Read the model definition and answer for the solid it produces. Units are mm, in the model's axes. A direction names the side the tool comes from. Coordinates: 2 decimals unless noted, no trailing zeros. Write each loop counter-clockwise with the first axis right and the second up, starting at its lowest first coordinate (ties: lowest second). Pieces come first, ordered by that corner, then holes. Notation, with made-up numbers: (11.25, 19) -> (31.25, 19) arc R24 ccw to (31.25, 55) -> close; hole circle Ø4 at (6, 33.5). An arc over 180 degrees is marked (long way). One line per item, written item: value. Start each with the question number.
1. For a pull along Y with two mould halves and no side action, classify faces 6 (the cylindrical face through (0, -15, 0)), 7 (the flat face through (0, -16.75, 0)), 8 (the flat face through (2, -7, -1.5)) as pulls with the +Y half, pulls with the -Y half, needs draft (parallel to the pull), parting line crosses it, or undercut.
2. For faces 1 (the flat face through (-5, 1.2, 1.14)), 2 (the cylindrical face through (0, -1.5, 0)), 3 (the cylindrical face through (7.03, 0.07, 1.5)), 4 (the flat face through (5, -1.2, -1.14)), 5 (the flat face through (-4, -9, 0)), determine the directions among +Z, -Z, +X, -X, +Y, -Y from which every point of the face is accessible in a straight line to the end or side of a thin tool.
3. Given P1, Ø3, axis at x = 7.5, y = -2, coming from the +Z side; P2, Ø2, axis at x = 0, y = -9.5, coming from the +Z side; P3, Ø1.5, axis at y = -12, z = -1, coming from the -X side, each flat-ended and moving along its own axis, determine where each tip first touches the part or whether it passes through.
4. Find section A-A, the plane x = 0. Write down the section's boundary in (y, z), and give its area (4 significant figures).
5. Consider line 1 along X through (y, z) = (-10.25, -0.2); line 2 along X through (y, z) = (-14, 1.05); line 3 along Y through (x, z) = (0.5, -0.3). Determine where each line is inside the solid, lowest interval first.
6. Find section B-B, the plane y = -12.25. Write down the section's boundary in (x, z), and give its area (3 significant figures).
```python
from build123d import *

# Parameters (mm, degrees)
BOSS_EXTRU_1_DEPTH = 1.5
ESQUISSE3_R        = 1.5
BOSS_EXTRU_2_DEPTH = 10


with BuildPart() as part:
    # Esquisse1 → Boss.-Extru.1 (new, symmetric)
    with BuildSketch(Plane.XY):
        with BuildLine():
            Line((-5, -1.5), (-4.585786438, -1.914213562))
            ThreePointArc((-4.585786438, -1.914213562), (-4.152240935, -2.56306026), (-4, -3.328427125))
            Line((-4, -3.328427125), (-4, -14.75))
            ThreePointArc((-4, -14.75), (-3.414213562, -16.164213562), (-2, -16.75))
            Line((-2, -16.75), (2, -16.75))
            ThreePointArc((2, -16.75), (3.414213562, -16.164213562), (4, -14.75))
            Line((4, -14.75), (4, -3.328427125))
            ThreePointArc((4, -3.328427125), (4.152240935, -2.56306026), (4.585786438, -1.914213562))
            Line((4.585786438, -1.914213562), (5, -1.5))
            Line((5, -1.5), (5, 1.5))
            Line((5, 1.5), (-5, 1.5))
            Line((-5, 1.5), (-5, -1.5))
        make_face()
        with BuildLine():
            Line((1.75, -3.25), (1.75, -13.25))
            ThreePointArc((1.75, -13.25), (0, -15), (-1.75, -13.25))
            Line((-1.75, -13.25), (-1.75, -3.25))
            ThreePointArc((-1.75, -3.25), (0, -1.5), (1.75, -3.25))
        make_face(mode=Mode.SUBTRACT)
    extrude(amount=BOSS_EXTRU_1_DEPTH, both=True)

    # Esquisse3 → Boss.-Extru.2 (add, symmetric)
    with BuildSketch(Plane(origin=(0, 0, 0), x_dir=(0, 0, -1), z_dir=(1, 0, 0))):
        Circle(ESQUISSE3_R)
    extrude(amount=BOSS_EXTRU_2_DEPTH, both=True)

    # Esquisse4 → Enlèvement de matière-Révolution1 (revolve, cut)
    with BuildSketch(Plane(origin=(0, 0, 0), x_dir=(1, 0, 0), z_dir=(0, 1, 0))):
        Polygon((-10, 1.5), (-9, 1.5), (-10, 1.232050808), align=None)
        Polygon((10, 1.232050808), (10, 1.5), (9, 1.5), align=None)
    revolve(axis=Axis((11, 0, 0), (-1, 0, 0)), mode=Mode.SUBTRACT)


solid = part.part
```
Answer block:
1. face 6: undercut
1. face 7: pulls with the -Y half
1. face 8: needs draft
2. face 1: +Z, -X, +Y
2. face 2: +Z, -Z
2. face 3: +X
2. face 4: -Z, +X, -Y
2. face 5: +Z, -Z, -X, -Y
3. P1: stops at z = 1.41
3. P2: passes through
3. P3: stops at x = -4
4. outline: (-16.75, -1.5) -> (-15, -1.5) -> (-15, 1.5) -> (-16.75, 1.5) -> close; (-1.5, -1.5) -> (1.5, -1.5) -> (1.5, 1.5) -> (-1.5, 1.5) -> close
4. area: 14.25 mm2
5. line 1: x = -4 to -1.75, 1.75 to 4
5. line 2: x = -4 to -1.58, 1.58 to 4
5. line 3: y = -16.75 to -14.93, -1.57 to 1.5
6. outline: (-4, -1.5) -> (-1.75, -1.5) -> (-1.75, 1.5) -> (-4, 1.5) -> close; (1.75, -1.5) -> (4, -1.5) -> (4, 1.5) -> (1.75, 1.5) -> close
6. area: 13.5 mm2
